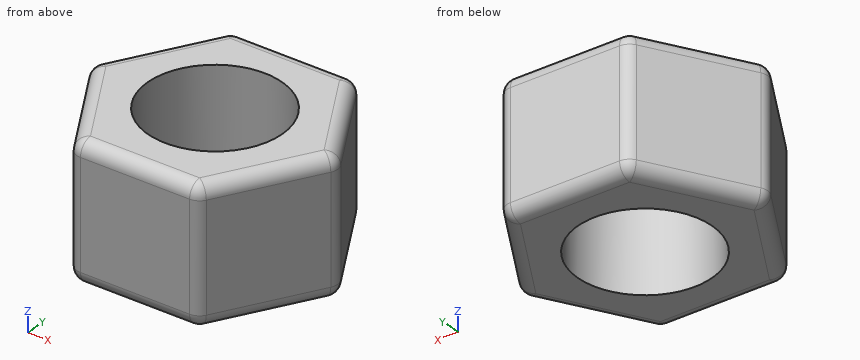
Autodesk Inventor part; units mm, degrees
ref_plane "YZ Plane" through (0, 0, 0) normal (1, 0, 0) x (0, 1, 0)
ref_plane "XZ Plane" through (0, 0, 0) normal (0, 1, 0) x (-1, 0, 0)
ref_plane "XY Plane" through (0, 0, 0) normal (0, 0, 1) x (1, 0, 0)
sketch "草图1" plane through (0, 0, 0) normal (0, 0, 1) x (1, 0, 0)
  line L0 (4.6188, -8) -> (-4.6188, -8)
  line L1 (-4.6188, -8) -> (-9.2376, 0)
  line L2 (-9.2376, 0) -> (-4.6188, 8)
  line L3 (-4.6188, 8) -> (4.6188, 8)
  line L4 (4.6188, 8) -> (9.2376, 0)
  line L5 (9.2376, 0) -> (4.6188, -8)
  line L6 (0, 0) -> (0, 8)
  circle A0 centre (0, 0) radius 5
  dimension "d0" = 16
  dimension "d1" = 10
extrude "拉伸1" add sketch "草图1" along normal blind 10
thread "螺纹1"
fillet "圆角1" radius 1 20 edges at (2.3094, 8, 10) (-2.3094, 8, 10) (-6.9282, 4, 10) (-6.9282, -4, 10) (0, -8, 10) (6.9282, -4, 10) (6.9282, 4, 10) (9.2376, 0, 5) (4.6188, 8, 5) (-4.6188, 8, 5) (-9.2376, 0, 5) (-4.6188, -8, 5) (4.6188, -8, 5) (6.9282, -4, 0) (6.9282, 4, 0) (2.3094, 8, 0) (-2.3094, 8, 0) (-6.9282, 4, 0) (-6.9282, -4, 0) (0, -8, 0)
properties part number "集肉斗固定螺帽"
Part model, mm, in its own coordinate system. Give positions to 0.01 mm unless a question says otherwise; leave off trailing zeros. Loops run counter-clockwise (first coordinate to the right, second up) from the corner with the lowest first, then second, coordinate; pieces in that order, holes last. Notation, with made-up numbers: M 37.5,38.25 L 49.5,38.25 A6 ccw 49.5,45.25 Z; hole C 70,61 d4. An arc over 180 degrees is marked long. Return JSON: item names as keys, results as strings.
1) Saw through at C-C, the plane x = 0. List the corners of the cut face in (y, z).
Calculated:
{"outline": "M -8,1 A1 ccw -7,0 L -5,0 L -5,10 L -7,10 A1 ccw -8,9 Z; M 5,0 L 7,0 A1 ccw 8,1 L 8,9 A1 ccw 7,10 L 5,10 Z"}
2) Saw through at B-B, the plane z = 3.5. List the corners of the cut face in (x, y).
Calculated:
{"outline": "M -8.95,-0.5 L -4.91,-7.5 A1 ccw -4.04,-8 L 4.04,-8 A1 ccw 4.91,-7.5 L 8.95,-0.5 A1 ccw 8.95,0.5 L 4.91,7.5 A1 ccw 4.04,8 L -4.04,8 A1 ccw -4.91,7.5 L -8.95,0.5 A1 ccw Z; hole C 0,0 d10"}
3) Flat gauge pin, fed straight in: pin 1 Ø1 at (x, y) = (-2, 2) entering from +Z. Where does the tip first touch, or does it go through?
Calculated:
{"pin 1": "passes through"}
4) Saw through at A-A, the plane x = -3. List the corners of the cut face in (y, z).
Calculated:
{"outline": "M -8,1 A1 ccw -7,0 L -4,0 L -4,10 L -7,10 A1 ccw -8,9 Z; M 4,0 L 7,0 A1 ccw 8,1 L 8,9 A1 ccw 7,10 L 4,10 Z"}
5) Drill centre lines: line 1 (Y direction, x = 0, z = 6.75); line 2 (X direction, y = 0, z = 6.25); line 3 (X direction, y = 2.25, z = 1). Where is each one in solid material? Low to high.
Calculated:
{"line 1": "y = -8 to -5, 5 to 8", "line 2": "x = -9.08 to -5, 5 to 9.08", "line 3": "x = -7.94 to -4.47, 4.47 to 7.94"}
